Could you check a few things on this model? Use its own coordinates, in mm. A direction names the side the tool comes from. Coordinates: 2 decimals unless noted, no trailing zeros. Write each loop counter-clockwise with the first axis right and the second up, starting at its lowest first coordinate (ties: lowest second). Pieces come first, ordered by that corner, then holes. Notation, with made-up numbers: M 14,23.25 L 45,23.25 A25 ccw 45,44.25 Z; hole C 87.25,-7.75 d6. An arc over 180 degrees is marked long. Answer as CSV lines item,"result". Start each with the question number.
Item 1: I'm going to push flat-ended pins straight in: P1, Ø8, axis at y = 10, z = 49.5, coming from the +X side; P2, Ø12, axis at x = 16, z = 12, coming from the +Y side; P3, Ø4.5, axis at y = 10, z = 85, coming from the +X side. Where does each tip first touch, or does it pass through?
Item 2: Suppose I cut it at B-B, the plane y = 10. Write out the boundary of the cut face in (x, z), and give its area (3 significant figures).
Item 3: Suppose I cut it at C-C, the plane x = 38. Write out the boundary of the cut face in (y, z), and give its area (3 significant figures).
Item 4: If I drill on line 1 along X through (y, z) = (8.5, 35.5); line 2 along Y through (x, z) = (2.3, 85), over which ranges is the centre line in solid material (lowest first)? Write a range as [from, to].
Item 5: On a 3-axis mill with a long thin cutter (end or side, diameter ignored), from which of +Z, -Z, +X, -X, +Y, -Y can I reach the whole of each face in a straight line? I mean faces 4 (the flat face through (3, 14, 49)), 5 (the cylindrical face through (1.479, 8.448, 11.976)). Say none if no direction works.
Item 6: Suppose I cut it at D-D, the plane z = 49.5. Write out the boundary of the cut face in (x, y).
Item 7: Suppose I cut it at A-A, the plane z = 85. Write out the boundary of the cut face in (x, y).
Item 8: We'd pull the mould along Z, two halves only. Please class faces 1 (the cylindrical face through (1.479, 9.023, 87.356)), 2 (the flat face through (25, 3, 49)), 3 (the flat face through (31.8, 2.6, -1)): +Z half, -Z half, draft (parallel to the pull), parting line (faces both ways), or undercut.
```python
from build123d import *

# Parameters (mm, degrees)
BASE_FLANGE1_DEPTH      = 100
BASE_FLANGE1_DEPTH_BACK = 1
FILLET1_R               = 5
CUT_EXTRUDE1_REACH      = 131.186
SKETCH2_R               = 19
CUT_EXTRUDE2_REACH      = 131.615
SKETCH3_R               = 2.55


# Sheet-metal steps are written as plain solids
with BuildPart() as part:
    # Sketch1 → Base-Flange1 (new, two sides: drawn at the far end of the back side and taken through both)
    with BuildSketch(Plane.XY.offset(-BASE_FLANGE1_DEPTH_BACK)):
        with BuildLine():
            Line((0, 20), (0, 3.7366))
            ThreePointArc((0, 3.7366), (1.094424801, 1.094424801), (3.7366, 0))
            Line((3.7366, 0), (80, 0))
            Line((80, 0), (80, 3))
            Line((80, 3), (3.7366, 3))
            ThreePointArc((3.7366, 3), (3.215745145, 3.215745145), (3, 3.7366))
            Line((3, 3.7366), (3, 20))
            Line((3, 20), (0, 20))
        make_face()
    extrude(amount=BASE_FLANGE1_DEPTH + BASE_FLANGE1_DEPTH_BACK)

    # Fillet1
    fillet1_edges = [part.edges().sort_by_distance(p)[0] for p in [
        (80, 1.5, -1),
        (80, 1.5, 100),
    ]]
    fillet(fillet1_edges, radius=FILLET1_R)

    # Sketch2 → Cut-Extrude1 (cut, up to next)
    with BuildSketch(Plane(origin=(0, 3, 0), x_dir=(1, 0, 0), z_dir=(0, 1, 0)), mode=Mode.PRIVATE) as cut_extrude1_sk1:
        with Locations(Location((48, -49, 0), (0, 0, 270))):
            Circle(SKETCH2_R)
    cut_extrude1_tool1 = extrude(cut_extrude1_sk1.sketch, amount=-CUT_EXTRUDE1_REACH, mode=Mode.PRIVATE) & part.part
    add(cut_extrude1_tool1.solids().sort_by_distance((48, 3, 49))[0], mode=Mode.SUBTRACT)

    # Sketch3 → Cut-Extrude2 (cut, up to next)
    with BuildSketch(Plane.ZY, mode=Mode.PRIVATE) as cut_extrude2_sk1:
        with Locations((14, 10)):
            Circle(SKETCH3_R)
    cut_extrude2_tool1 = extrude(cut_extrude2_sk1.sketch, amount=-CUT_EXTRUDE2_REACH, mode=Mode.PRIVATE) & part.part
    # Sketch3 → Cut-Extrude2 (cut, up to next)
    with BuildSketch(Plane.ZY, mode=Mode.PRIVATE) as cut_extrude2_sk2:
        with Locations((49.5, 10)):
            Circle(SKETCH3_R)
    cut_extrude2_tool2 = extrude(cut_extrude2_sk2.sketch, amount=-CUT_EXTRUDE2_REACH, mode=Mode.PRIVATE) & part.part
    # Sketch3 → Cut-Extrude2 (cut, up to next)
    with BuildSketch(Plane.ZY, mode=Mode.PRIVATE) as cut_extrude2_sk3:
        with Locations((85, 10)):
            Circle(SKETCH3_R)
    cut_extrude2_tool3 = extrude(cut_extrude2_sk3.sketch, amount=-CUT_EXTRUDE2_REACH, mode=Mode.PRIVATE) & part.part
    add(cut_extrude2_tool1.solids().sort_by_distance((0, 10, 14))[0], mode=Mode.SUBTRACT)
    add(cut_extrude2_tool2.solids().sort_by_distance((0, 10, 49.5))[0], mode=Mode.SUBTRACT)
    add(cut_extrude2_tool3.solids().sort_by_distance((0, 10, 85))[0], mode=Mode.SUBTRACT)


solid = part.part
```
Ans:
1,P1,"stops at x = 3"
1,P2,"stops at y = 3"
1,P3,"passes through"
2,outline,"M 0,-1 L 3,-1 L 3,11.45 L 0,11.45 Z; M 0,16.55 L 3,16.55 L 3,46.95 L 0,46.95 Z; M 0,52.05 L 3,52.05 L 3,82.45 L 0,82.45 Z; M 0,87.55 L 3,87.55 L 3,100 L 0,100 Z"
2,area,"257 mm^2"
3,outline,"M 0,-1 L 3,-1 L 3,32.84 L 0,32.84 Z; M 0,65.16 L 3,65.16 L 3,100 L 0,100 Z"
3,area,"206 mm^2"
4,line 1,"x = [0, 3]"
4,line 2,"y = [0.29, 7.45], [12.55, 20]"
5,face 4,"+Z, -Z, +X, +Y"
5,face 5,"+X, -X"
6,outline,"M 0,3.74 A3.74 ccw 3.74,0 L 29.01,0 L 29.01,3 L 3.74,3 A0.74 cw 3,3.74 L 3,7.45 L 0,7.45 Z; M 0,12.55 L 3,12.55 L 3,20 L 0,20 Z; M 66.99,0 L 80,0 L 80,3 L 66.99,3 Z"
7,outline,"M 0,3.74 A3.74 ccw 3.74,0 L 80,0 L 80,3 L 3.74,3 A0.74 cw 3,3.74 L 3,7.45 L 0,7.45 Z; M 0,12.55 L 3,12.55 L 3,20 L 0,20 Z"
8,face 1,"undercut"
8,face 2,"draft"
8,face 3,"-Z half"
